```python
from build123d import *

# Parameters (mm, degrees)
SKETCH2_W           = 133.35
SKETCH2_H           = 160.866666666
SKETCH2_W_2         = 107.95
SKETCH2_H_2         = 135.466666666
BOSS_EXTRUDE1_DEPTH = 12.7
CUT_EXTRUDE1_DEPTH  = 6.35
CHAMFER4_SIZE       = 3.81
CHAMFER1_SIZE       = 0.635
CHAMFER2_SIZE       = 3.175
SKETCH4_W           = 8.89
SKETCH4_H           = 11.43
CUT_EXTRUDE2_DEPTH  = 10.16
SKETCH5_W           = 8.89
SKETCH5_H           = 11.43
CUT_EXTRUDE3_DEPTH  = 10.16


with BuildPart() as part:
    # Sketch2 → Boss-Extrude1 (new body)
    with BuildSketch(Plane(origin=(0, 0, 0), x_dir=(1, 0, 0), z_dir=(0, 1, 0))):
        Rectangle(SKETCH2_W, SKETCH2_H)
        Rectangle(SKETCH2_W_2, SKETCH2_H_2, mode=Mode.SUBTRACT)
    extrude(amount=BOSS_EXTRUDE1_DEPTH)

    # Sketch3 → Cut-Extrude1 (cut)
    with BuildSketch(Plane.XZ):
        Polygon((-57.15, 76.2), (-60.325, 73.025), (-63.5, 76.2), (-60.325, 79.375), align=None)
        Polygon((57.15, 76.2), (53.975, 73.025), (50.8, 76.2), (53.975, 79.375), align=None)
        Polygon((57.15, -76.2), (53.975, -79.375), (50.8, -76.2), (53.975, -73.025), align=None)
        Polygon((-57.15, -76.2), (-60.325, -79.375), (-63.5, -76.2), (-60.325, -73.025), align=None)
    extrude(amount=-CUT_EXTRUDE1_DEPTH, mode=Mode.SUBTRACT)

    # Chamfer4
    chamfer4_edges = [part.edges().sort_by_distance(p)[0] for p in [
        (0, 12.7, -80.433333333),
        (0, 12.7, 80.433333333),
    ]]
    chamfer(chamfer4_edges, length=CHAMFER4_SIZE)

    # Chamfer1
    chamfer1_edges = [part.edges().sort_by_distance(p)[0] for p in [
        (-58.7375, 6.35, -74.6125),
        (-58.7375, 6.35, -77.7875),
        (-61.9125, 6.35, -77.7875),
        (-61.9125, 6.35, -74.6125),
        (-58.7375, 0, -74.6125),
        (-61.9125, 0, -74.6125),
        (-61.9125, 0, -77.7875),
        (-58.7375, 0, -77.7875),
        (55.5625, 6.35, -74.6125),
        (55.5625, 6.35, -77.7875),
        (52.3875, 6.35, -77.7875),
        (52.3875, 6.35, -74.6125),
        (55.5625, 0, -74.6125),
        (52.3875, 0, -74.6125),
        (52.3875, 0, -77.7875),
        (55.5625, 0, -77.7875),
        (55.5625, 6.35, 77.7875),
        (55.5625, 6.35, 74.6125),
        (52.3875, 6.35, 74.6125),
        (52.3875, 6.35, 77.7875),
        (55.5625, 0, 77.7875),
        (52.3875, 0, 77.7875),
        (52.3875, 0, 74.6125),
        (55.5625, 0, 74.6125),
        (-58.7375, 6.35, 77.7875),
        (-58.7375, 6.35, 74.6125),
        (-61.9125, 6.35, 74.6125),
        (-61.9125, 6.35, 77.7875),
        (-58.7375, 0, 77.7875),
        (-61.9125, 0, 77.7875),
        (-61.9125, 0, 74.6125),
        (-58.7375, 0, 74.6125),
    ]]
    chamfer(chamfer1_edges, length=CHAMFER1_SIZE)

    # Chamfer2
    chamfer2_edges = [part.edges().sort_by_distance(p)[0] for p in [
        (53.975, 0, 0),
        (0, 0, -67.733333333),
        (0, 0, 67.733333333),
    ]]
    chamfer(chamfer2_edges, length=CHAMFER2_SIZE)

    # Sketch4 → Cut-Extrude2 (cut)
    with BuildSketch(Plane.XY.offset(80.433333333)):
        with Locations((38.0365, 6.985)):
            Rectangle(SKETCH4_W, SKETCH4_H)
    extrude(amount=-CUT_EXTRUDE2_DEPTH, mode=Mode.SUBTRACT)

    # Sketch5 → Cut-Extrude3 (cut)
    with BuildSketch(Plane(origin=(0, 0, -80.433333333), x_dir=(-1, 0, 0), z_dir=(0, 0, -1))):
        with Locations((-38.0365, 6.985)):
            Rectangle(SKETCH5_W, SKETCH5_H)
    extrude(amount=-CUT_EXTRUDE3_DEPTH, mode=Mode.SUBTRACT)


solid = part.part
```
The listing builds one solid part. Answer for the finished solid, in the listing's coordinates (mm). A direction names the side the tool comes from. Coordinates: 2 decimals unless noted, no trailing zeros. Loops run counter-clockwise (first coordinate to the right, second up) from the corner with the lowest first, then second, coordinate; pieces in that order, holes last. Notation, with made-up numbers: (60, 78) - (111, 78) arc R14 cw to (111, 96) - close; hole circle Ø10 at (88, 59.25). An arc over 180 degrees is marked (long way). Use a Markdown table: item, result. Add a question column.
1) Find the intervals of material crossed by line 1 (X direction, y = 9.5, z = -8) (3 decimals); line 2 (Z direction, x = 41, y = 7.5); line 3 (X direction, y = 5.75, z = -71) (1 decimal), in increasing order.
2) For faces 1 (the flat face through (-55, 12.7, 0)), 2 (the flat face through (42.482, 7, -75)), 3 (the flat face through (-61.7, 6, 74.8)), determine the directions among +Z, -Z, +X, -X, +Y, -Y from which every point of the face is accessible in a straight line to the end or side of a thin tool.
3) The part is cut by section B-B, the plane x = 8. Give the vertices of the cut face in (y, z) (3 decimals).
4) Given pin 1 (2.5 mm diameter, centred on x = 53.5, z = 76.5, fed in from -Y); pin 2 (2.5 mm diameter, centred on x = -60, z = 77, fed in from -Y); pin 3 (4.5 mm diameter, centred on x = 37, y = 6, fed in from -Z), each flat-ended and moving along its own axis, determine where each tip first touches the part or whether it passes through.
5) The mould has two halves that part along X. Classify faces 4 (the flat face through (66.675, 6, 1)), 5 (the flat face through (-17.244, 10.822, 78.502)), 6 (the flat face through (55.812, 0.322, 74.42)), 7 (the flat face through (-58.545, 0.322, -74.363)): released by +X, released by -X, zero draft, split by the parting line, or undercut.
6) The part is cut by section A-A, the plane z = 65.5. Give the vertices of the cut face in (x, y) (3 decimals), and give its area (3 significant figures).
Here are the results:
| question | item | result |
|---|---|---|
| 1 | line 1 | x = -66.675 to -53.975, 53.975 to 66.675 |
| 1 | line 2 | z = -70.27 to -67.73, 67.73 to 70.27 |
| 1 | line 3 | x = -66.7 to 33.6, 42.5 to 66.7 |
| 2 | face 1 | +Z, -Z, +X, -X, +Y |
| 2 | face 2 | -Z, +Y |
| 2 | face 3 | -Y |
| 3 | outline | (0, -80.433) - (8.89, -80.433) - (12.7, -76.623) - (12.7, -67.733) - (3.175, -67.733) - (0, -70.908) - close; (0, 70.908) - (3.175, 67.733) - (12.7, 67.733) - (12.7, 76.623) - (8.89, 80.433) - (0, 80.433) - close |
| 4 | pin 1 | stops at y = 6.16 |
| 4 | pin 2 | stops at y = 5.91 |
| 4 | pin 3 | stops at z = -70.27 |
| 5 | face 4 | released by +X |
| 5 | face 5 | zero draft |
| 5 | face 6 | undercut |
| 5 | face 7 | undercut |
| 6 | outline | (-66.675, 0) - (-53.975, 0) - (-53.975, 12.7) - (-66.675, 12.7) - close; (53.975, 3.175) - (57.15, 0) - (66.675, 0) - (66.675, 12.7) - (53.975, 12.7) - close |
| 6 | area | 318 mm^2 |
